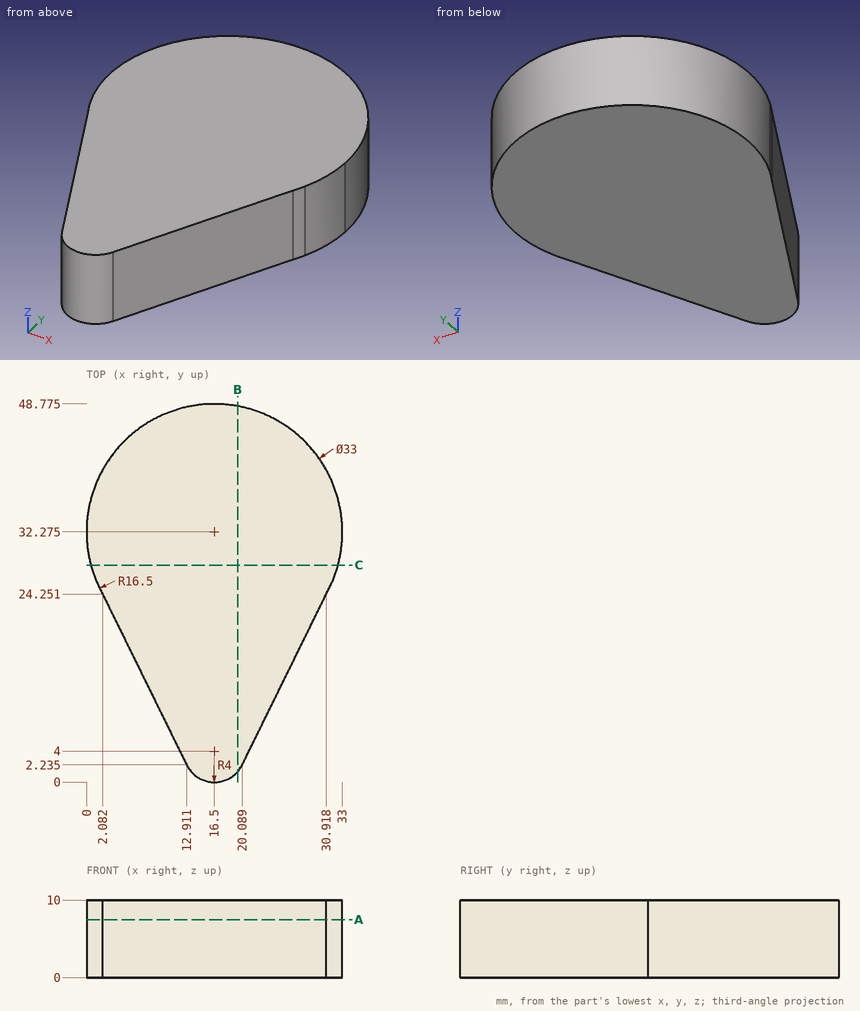
Source: three-view drawing plus pictorial views. Frame: mm from the lowest corner of the part. Give positions to 0.01 mm unless a question says otherwise; leave off trailing zeros. Order: outer loops, then holes, each group sorted by start corner. A loop starts at its lowest first (then second) coordinate and runs counter-clockwise, first axis right, second up. Notation, with made-up numbers: (-18, 64) -> (40, 64) arc R19 ccw to (40, 79) -> close; hole circle Ø6 at (89, 65.25). An arc over 180 degrees is marked (long way). Use a Markdown table: item, result.
Q1. Material intervals for line 1 (X direction, y = 13.5, z = 2); line 2 (Y direction, x = 21.5, z = 6.5) (1 decimal); line 3 (X direction, y = 30.5, z = 2.5) (1 decimal), sorted ascending. Write a range as [from, to].
A:
| item | result |
|---|---|
| line 1 | [7.37, 25.63] |
| line 2 | [5.1, 48] |
| line 3 | [0.1, 32.9] |
Q2. Section C-C (y = 28). Return the cut outline in (x, z).
A:
| item | result |
|---|---|
| outline | (0.56, 0) -> (32.44, 0) -> (32.44, 10) -> (0.56, 10) -> close |
Q3. First-contact query: P1, Ø4, axis at x = 13, z = 7, coming from the +Y side; P2, Ø2, axis at x = 8, z = 9, coming from the +Y side; P3, Ø4, axis at x = 15.5, z = 8, coming from the -Y side; P4, Ø5, axis at x = 29.5, z = 5.5, coming from the -Y side (1 decimal). Flat tips, straight axial feed; report the tip coordinate or a pass-through.
A:
| item | result |
|---|---|
| P1 | y = 48.71 |
| P2 | y = 46.97 |
| P3 | y = 0 |
| P4 | y = 16.3 |
Q4. Section B-B (x = 19.5). Return the cut outline in (y, z) (1 decimal).
A:
| item | result |
|---|---|
| outline | (1.4, 0) -> (48.5, 0) -> (48.5, 10) -> (1.4, 10) -> close |
Q5. Section A-A (z = 7.5). Return the cut outline in (x, y) (1 decimal).
A:
| item | result |
|---|---|
| outline | (2.1, 24.3) -> (12.9, 2.2) arc R4 ccw to (20.1, 2.2) -> (30.9, 24.3) arc R16.5 ccw (long way) to start |
